from build123d import *

# Parameters (mm, degrees)
SKETCH_1_W             = 63.5
SKETCH_1_H             = 24
EXTRUDE_1_DEPTH        = 5.5
SKETCH_2_W             = 35
SKETCH_2_H             = 3
CUT_EXTRUDE_2_DEPTH    = 24
HOLE_WIZARD_M3_1_D     = 2.5
HOLE_WIZARD_M3_1_DEPTH = 7.5
HOLE_WIZARD_M3_1_TIP   = 0.751075774
CHAMFER_1_SIZE         = 0.5
CHAMFER_2_SIZE         = 0.5
CHAMFER_3_SIZE         = 5.5
SKETCH_7_W             = 20
SKETCH_7_H             = 18.5
EXTRUDE_1_2_DEPTH      = 3
SKETCH_8_R             = 3.5
CUT_EXTRUDE_1_DEPTH    = 3
SKETCH_9_R             = 2.25
CUT_EXTRUDE_2_2_DEPTH  = 87
CUT_EXTRUDE_4_DEPTH    = 10
FILLET_1_R             = 3
CHAMFER_5_SIZE         = 0.2
FILLET_3_R             = 2
SKETCH_11_R            = 1.25
CUT_EXTRUDE_5_DEPTH    = 96
CHAMFER_6_SIZE         = 0.1
SKETCH_12_W            = 35
SKETCH_12_H            = 24
EXTRUDE_2_DEPTH        = 3
SKETCH_13_W            = 36
SKETCH_13_H            = 24
CUT_EXTRUDE_6_DEPTH    = 3
CUT_EXTRUDE_7_DEPTH    = 0.5


with BuildPart() as part:
    # 草图1 → Extrude 1 (new body)
    with BuildSketch(Plane.XY):
        Rectangle(SKETCH_1_W, SKETCH_1_H)
    extrude(amount=EXTRUDE_1_DEPTH)

    # 草图2 → Cut-Extrude 2 (cut)
    with BuildSketch(Plane.XZ.offset(12)):
        with Locations((0, 1.5)):
            Rectangle(SKETCH_2_W, SKETCH_2_H)
    extrude(amount=-CUT_EXTRUDE_2_DEPTH, mode=Mode.SUBTRACT)

    # M3 螺纹孔1
    with Locations(Plane(origin=(22.5, 8, 0), x_dir=(-1, 0, 0), z_dir=(0, 0, -1))):
        with Locations((0, 0), (0, -15), (45, -15), (45, 0)):
            Hole(HOLE_WIZARD_M3_1_D / 2, depth=HOLE_WIZARD_M3_1_DEPTH)
            with Locations((0, 0, -(HOLE_WIZARD_M3_1_DEPTH + HOLE_WIZARD_M3_1_TIP / 2))):  # 118° drill point
                Cone(0, HOLE_WIZARD_M3_1_D / 2, HOLE_WIZARD_M3_1_TIP, mode=Mode.SUBTRACT)

    # 倒角1
    chamfer_1_edges = [part.edges().sort_by_distance(p)[0] for p in [
        (-23.75, 8, 0),
        (-23.75, -7, 0),
        (21.25, -7, 0),
        (21.25, 8, 0),
    ]]
    chamfer(chamfer_1_edges, length=CHAMFER_1_SIZE)

    # 倒角2
    chamfer_2_edges = [part.edges().sort_by_distance(p)[0] for p in [
        (-23.75, 8, 5.5),
        (-23.75, -7, 5.5),
        (21.25, -7, 5.5),
        (21.25, 8, 5.5),
    ]]
    chamfer(chamfer_2_edges, length=CHAMFER_2_SIZE)

    # 倒角3
    chamfer_3_edges = [part.edges().sort_by_distance(p)[0] for p in [
        (31.75, -12, 2.75),
        (-31.75, -12, 2.75),
    ]]
    chamfer(chamfer_3_edges, length=CHAMFER_3_SIZE)

    # 草图7 → Extrude 1 2 (add)
    with BuildSketch(Plane(origin=(31.75, 0, 0), x_dir=(0, 0, -1), z_dir=(1, 0, 0))):
        with Locations((-10, 2.75)):
            Rectangle(SKETCH_7_W, SKETCH_7_H)
    extrude_1_2 = extrude(amount=EXTRUDE_1_2_DEPTH)

    # 草图8 → 切除-拉伸1 (cut)
    with BuildSketch(Plane(origin=(34.75, 0, 0), x_dir=(0, 0, -1), z_dir=(1, 0, 0))):
        with Locations((-7, 2.95)):
            Circle(SKETCH_8_R)
    cut_extrude_1 = extrude(amount=-CUT_EXTRUDE_1_DEPTH, mode=Mode.SUBTRACT)

    # 草图9 → Cut-Extrude 2 2 (cut)
    with BuildSketch(Plane(origin=(34.75, 0, 0), x_dir=(0, 0, -1), z_dir=(1, 0, 0))):
        with Locations((-15.5, -3.25)):
            Circle(SKETCH_9_R)
    cut_extrude_2_2 = extrude(amount=-CUT_EXTRUDE_2_2_DEPTH, mode=Mode.SUBTRACT)

    # 草图10 → 切除-拉伸4 (cut)
    with BuildSketch(Plane(origin=(31.75, 0, 0), x_dir=(0, 0, -1), z_dir=(1, 0, 0))):
        Polygon((-20, 1.465133344), (-20, 12), (-5.5, 12), align=None)
    cut_extrude_4 = extrude(amount=CUT_EXTRUDE_4_DEPTH, mode=Mode.SUBTRACT)

    # 镜向2: Extrude 1 2, 切除-拉伸1, Cut-Extrude 2 2, 切除-拉伸4 across plane
    add(extrude_1_2.mirror(Plane(origin=(0, 0, 0), x_dir=(0, 0, 1), z_dir=(1, 0, 0))))
    add(cut_extrude_1.mirror(Plane(origin=(0, 0, 0), x_dir=(0, 0, 1), z_dir=(1, 0, 0))), mode=Mode.SUBTRACT)
    add(cut_extrude_2_2.mirror(Plane(origin=(0, 0, 0), x_dir=(0, 0, 1), z_dir=(1, 0, 0))), mode=Mode.SUBTRACT)
    add(cut_extrude_4.mirror(Plane(origin=(0, 0, 0), x_dir=(0, 0, 1), z_dir=(1, 0, 0))), mode=Mode.SUBTRACT)

    # 圆角1
    fillet_1_edges = [part.edges().sort_by_distance(p)[0] for p in [
        (33.25, -6.5, 20),
        (33.25, 1.465133344, 20),
        (-33.25, 1.465133344, 20),
        (-33.25, -6.5, 20),
    ]]
    fillet(fillet_1_edges, radius=FILLET_1_R)

    # 倒角5
    chamfer_5_edges = [part.edges().sort_by_distance(p)[0] for p in [
        (34.75, 2.95, 10.5),
        (34.75, -3.25, 17.75),
        (-34.75, 2.95, 10.5),
        (-34.75, -3.25, 17.75),
    ]]
    chamfer(chamfer_5_edges, length=CHAMFER_5_SIZE)

    # 圆角3
    fillet_3_edges = [part.edges().sort_by_distance(p)[0] for p in [
        (0, -12, 5.5),
    ]]
    fillet(fillet_3_edges, radius=FILLET_3_R)

    # 草图11 → 切除-拉伸5 (cut)
    with BuildSketch(Plane.ZY.offset(34.75)):
        with Locations((11.2, -4.6)):
            Circle(SKETCH_11_R)
    extrude(amount=-CUT_EXTRUDE_5_DEPTH, mode=Mode.SUBTRACT)

    # 倒角6
    chamfer_6_edges = [part.edges().sort_by_distance(p)[0] for p in [
        (34.75, -4.6, 9.95),
        (-34.75, -4.6, 9.95),
    ]]
    chamfer(chamfer_6_edges, length=CHAMFER_6_SIZE)

    # 草图12 → 凸台-拉伸2 (add)
    with BuildSketch(Plane(origin=(0, 0, 3), x_dir=(-1, 0, 0), z_dir=(0, 0, -1))):
        Rectangle(SKETCH_12_W, SKETCH_12_H)
    extrude(amount=EXTRUDE_2_DEPTH)

    # 草图13 → 切除-拉伸6 (cut)
    with BuildSketch(Plane(origin=(0, 0, 0), x_dir=(-1, 0, 0), z_dir=(0, 0, -1))):
        Rectangle(SKETCH_13_W, SKETCH_13_H)
    extrude(amount=-CUT_EXTRUDE_6_DEPTH, mode=Mode.SUBTRACT)

    # 草图14 → 切除-拉伸7 (cut)
    with BuildSketch(Plane.XY.offset(5.5)):
        Polygon((31.75, -6.5), (25.25, -13), (-25.25, -13), (-31.75, -6.5), (-31.75, 12), (31.75, 12), align=None)
    extrude(amount=-CUT_EXTRUDE_7_DEPTH, mode=Mode.SUBTRACT)


solid = part.part
Geometry: final body of the model. Coordinates: model frame, mm. A direction names the side the tool comes from. Give positions to 0.01 mm unless a question says otherwise; leave off trailing zeros. Order: outer loops, then holes, each group sorted by start corner. A loop starts at its lowest first (then second) coordinate and runs counter-clockwise, first axis right, second up. Notation, with made-up numbers: (57, 33.25) -> (93, 33.25) arc R28 cw to (93, 59.25) -> close; hole circle Ø3 at (-11.75, 19.25). An arc over 180 degrees is marked (long way). Answer as a JSON object with one key per item and string values.
Q1. Section A-A (z = 2.25). Output: boundary loops of the cut face in (x, y).
Entries:
{"outline": "(-34.75, -6.5) -> (-31.75, -6.5) -> (-26.25, -12) -> (-18, -12) -> (-18, 12) -> (-34.75, 12) -> close; (18, -12) -> (26.25, -12) -> (31.75, -6.5) -> (34.75, -6.5) -> (34.75, 12) -> (18, 12) -> close; hole circle Ø2.5 at (-22.5, -7); hole circle Ø2.5 at (-22.5, 8); hole circle Ø2.5 at (22.5, -7); hole circle Ø2.5 at (22.5, 8)"}
Q2. Access query for faces 1 (the flat face through (-18, 0, 1)), 2 (the cylindrical face through (23.655, 7.521, 2.781)), 3 (the flat face through (31.75, 1, 13)). Directions: +Z, -Z, +X, -X, +Y, -Y. A direction counts if a zero-diameter tool reaches every point of the face in a straight line with its end or side. Return the directions, or none.
Entries:
{"face 1": "-Z, +Y, -Y", "face 2": "+Z, -Z", "face 3": "+Z, +Y, -Y"}
Q3. Section C-C (z = 15.5). Output: boundary loops of the cut face in (x, y).
Entries:
{"outline": "(-34.75, -6.5) -> (-31.75, -6.5) -> (-31.75, -5.5) -> (-34.55, -5.5) -> (-34.75, -5.7) -> close; (-34.75, -0.8) -> (-34.55, -1) -> (-31.75, -1) -> (-31.75, 4.73) -> (-34.75, 4.73) -> close; (31.75, -6.5) -> (34.75, -6.5) -> (34.75, -5.7) -> (34.55, -5.5) -> (31.75, -5.5) -> close; (31.75, -1) -> (34.55, -1) -> (34.75, -0.8) -> (34.75, 4.73) -> (31.75, 4.73) -> close"}
Q4. Section D-D (y = -10). Output: boundary loops of the cut face in (x, z), plus the area to 4 significant figures.
Entries:
{"outline": "(-28.25, 0) -> (-18, 0) -> (-18, 3) -> (18, 3) -> (18, 0) -> (28.25, 0) -> (28.25, 5) -> (-28.25, 5) -> close", "area": "174.5 mm^2"}
Q5. First-contact query: pin 1 (8 mm diameter, centred on y = 2.95, z = 7, fed in from +X); pin 2 (3.5 mm diameter, centred on x = 32.5, z = 12.5, fed in from -Y); pin 3 (12 mm diameter, centred on x = -7, y = -2.5, fed in from -Z). Flat tips, straight axial feed; report the tip coordinate or a pass-through.
Entries:
{"pin 1": "stops at x = 34.75", "pin 2": "stops at y = -6.5", "pin 3": "stops at z = 3"}
Q6. Draft query along X for faces 4 (the cylindrical face through (23.655, -7.479, 2.781)), 5 (the flat face through (31.75, 3, 4)), 6 (the cylindrical face through (-33.27, -5.6, 19.14)), 7 (the flat face through (0, 0, 3)). Return one class per face: released by +X, released by -X, zero draft, split by the parting line, or undercut.
Entries:
{"face 4": "undercut", "face 5": "released by +X", "face 6": "zero draft", "face 7": "undercut"}
Q7. Material intervals for probe 1 along Y at (x, z) = (22.5, 2.1); probe 2 along Y at (x, z) = (-22.5, 4.1); probe 3 along X at (y, z) = (3, 13.5), sorted ascending.
Entries:
{"probe 1": "y = -12 to -8.25, -5.75 to 6.75, 9.25 to 12", "probe 2": "y = -11.91 to -8.25, -5.75 to 6.75, 9.25 to 12", "probe 3": "x = -34.75 to -31.75, 31.75 to 34.75"}
Q8. Section B-B (x = 22.5). Output: boundary loops of the cut face in (y, z).
Entries:
{"outline": "(-12, 0) -> (-8.75, 0) -> (-8.25, 0.5) -> (-8.25, 5) -> (-11.32, 5) arc R2 ccw to (-12, 3.5) -> close; (-5.75, 0.5) -> (-5.25, 0) -> (6.25, 0) -> (6.75, 0.5) -> (6.75, 5) -> (-5.75, 5) -> close; (9.25, 0.5) -> (9.75, 0) -> (12, 0) -> (12, 5) -> (9.25, 5) -> close"}
